Check sheet for the modelled part. Datum: model origin and axes. Units: mm. Coordinates: 2 decimals unless noted, no trailing zeros. Order: outer loops, then holes, each group sorted by start corner. A loop starts at its lowest first (then second) coordinate and runs counter-clockwise, first axis right, second up. Notation, with made-up numbers: M -34,54.25 L 21,54.25 A20 cw 21,83.25 Z; hole C -40,4 d6. An arc over 180 degrees is marked long. Answer in a Markdown table with one row per item. Add a question column.
from build123d import *

# Parameters (mm, degrees)
F0_R     = 85
F2_R     = 0.5
F4_R     = 105.9677495378
F5_DEPTH = 1


# Not quite as in the source:
# - a fillet or chamfer that OpenCascade refuses, or shapes differently, is made with other operations: its cross-section is extruded or revolved along the edge and cut away or added


with BuildPart() as f3:
    # F0 (on Top) → F3 section 0
    with BuildSketch(Plane.XY):
        Circle(F0_R)
    # F2 (on offset) → F3 section 1
    with BuildSketch(Plane.XY.offset(1400)):
        Circle(F2_R)
    loft()

    # F4 (on Top) → F5 (join)
    with BuildSketch(Plane.XY):
        Circle(F4_R)
    extrude(amount=F5_DEPTH)

    # F6: fillet of radius 50 on 1 edges, made by hand


with BuildPart() as f6_tool2:
    # F6_s3 → F6_t4 (revolve)
    with BuildSketch(Plane.XZ):
        with BuildLine():
            ThreePointArc((105.9675375029, 0.9996608228), (89.4883112296, 17.8541588617), (82.5620399387, 40.3855984233))
            Line((82.5620399387, 40.3855984233), (77.5709757484, 40.0843520489))
            ThreePointArc((77.5709757484, 40.0843520489), (78.7599768444, 20.3915648868), (79.9485786669, 0.6987536257))
            Line((79.9485786669, 0.6987536257), (84.9396428571, -4.0001471107))
            ThreePointArc((84.9396428571, -4.0001471107), (95.45359018, -4.0001471107), (103.3170230691, -3.2401793116))
            Line((103.3170230691, -3.2401793116), (105.9675375029, 0.9996608228))
        make_face()
    revolve(axis=Axis((0, 0, 1), (0, 0, 1)))

    split(bisect_by=Plane.XY, keep=Keep.TOP)


with BuildPart() as f3_1:
    add(f3.part)

    # F6_t1: union F6_tool2
    add(f6_tool2.part)


solid = f3_1.part
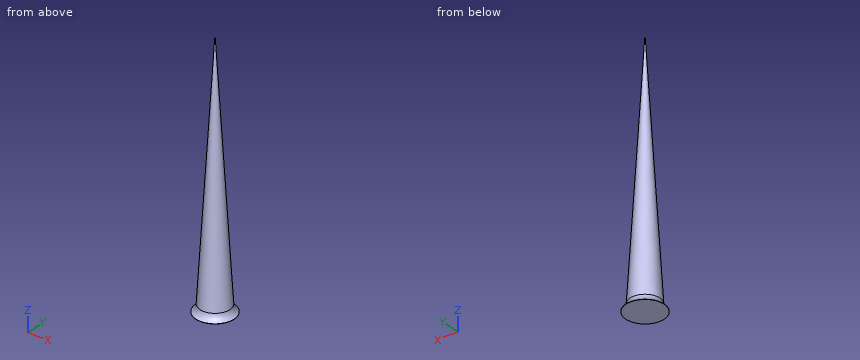
1. Section check B-B on z = 309. Enter the section's corners in (x, y), then the cut area to 3 significant figures.
2. Section check A-A on z = 1148.5. Enter the section's corners in (x, y).
3. Go/stop test with flat-tipped pins: pin 1 Ø1.5 at (x, y) = (-57, -28.5) entering from -Z; pin 2 Ø3 at (x, y) = (-42, 80) entering from +Z; pin 3 Ø4 at (y, z) = (-12.5, 512.5) entering from +X; pin 4 Ø1.5 at (x, y) = (82.5, 55) entering from +Z. Record where each tip stops, or that it passes through.
4. Scan lines: line 1 (Z direction, x = 72.5, y = -58); line 2 (Z direction, x = 44, y = 77.5); line 3 (Y direction, x = 2.5, z = 1219.5). Record each from-to range of solid material in increasing order.
Result sheet:
| question | item | result |
|---|---|---|
| 1 | outline | C 0,0 d132.7 |
| 1 | area | 13,800 mm^2 |
| 2 | outline | C 0,0 d31.36 |
| 3 | pin 1 | z = 0 |
| 3 | pin 2 | z = 18.95 |
| 3 | pin 3 | x = 53.06 |
| 3 | pin 4 | z = 6.8 |
| 4 | line 1 | 0 to 12.91 |
| 4 | line 2 | 0 to 18.49 |
| 4 | line 3 | -11.12 to 11.12 |
